```python
from build123d import *

# Parameters (mm, degrees)
F1_DEPTH = 63.5
F0_W     = 23.120732
F0_H     = 17.456719
F2_DEPTH = 25.4
F3_DEPTH = 7.9375
F5_R     = 6.35


with BuildPart() as f1:
    # F0 (on Front) → F1 (new body, symmetric)
    with BuildSketch(Plane.XZ):
        Polygon((23.818281, 9.525), (-41.275, 9.525), (-41.275, -9.525), (41.275, -9.525), (41.275, 9.525), align=None)
    extrude(amount=F1_DEPTH, both=True)

    # F0 (on Front) → F2 (join, symmetric)
    with BuildSketch(Plane.XZ):
        with Locations((71.885366, 61.128559)):
            Rectangle(F0_W, F0_H)
        with BuildLine():
            Line((23.818281, 36.5252), (23.818281, 9.525))
            Line((23.818281, 9.525), (41.275, 9.525))
            Line((41.275, 9.525), (41.275, 36.5252))
            ThreePointArc((41.275, 36.5252), (45.92468, 47.75052), (57.15, 52.4002))
            Line((57.15, 52.4002), (60.325, 52.4002))
            Line((60.325, 52.4002), (60.325, 69.856919))
            Line((60.325, 69.856919), (57.15, 69.856919))
            ThreePointArc((57.15, 69.856919), (33.580915, 60.094285), (23.818281, 36.5252))
        make_face()
    extrude(amount=F2_DEPTH, both=True)

    # F0 (on Front) → F3 (join, symmetric)
    with BuildSketch(Plane.XZ):
        with BuildLine():
            add(Edge.make_bspline(
                [(-41.275, 9.525), (-34.914378, 38.415078), (20.892713, 70.120394), (57.15, 69.856919)],
                knots=[0, 0, 0, 0, 115.44445, 115.44445, 115.44445, 115.44445], degree=3))
            Line((-41.275, 9.525), (23.818281, 9.525))
            Line((23.818281, 9.525), (23.818281, 36.5252))
            ThreePointArc((23.818281, 36.5252), (33.580915, 60.094285), (57.15, 69.856919))
        make_face()
    extrude(amount=F3_DEPTH, both=True)

    # F0 (on Front) → F4 (revolve)
    with BuildSketch(Plane.XZ):
        Polygon((83.445732, 76.2), (83.445732, 69.856919), (83.445732, 52.4002), (83.445732, 47.625), (111.125, 47.625), (111.125, 76.2), align=None)
    revolve(axis=Axis((83.445732, 0, 61.9125), (0, 0, 1)))

    # F5
    f5_edges = [f1.edges().sort_by_distance(p)[0] for p in [
        (-41.275, -63.5, 0),
        (41.275, -63.5, 0),
        (41.275, 63.5, 0),
        (-41.275, 63.5, 0),
    ]]
    fillet(f5_edges, radius=F5_R)


solid = f1.part
```
The model under review builds one solid part; all positions refer to its coordinate system, in mm. A direction names the side the tool comes from. Round coordinates to 2 decimals unless told otherwise and drop trailing zeros. Order: outer loops, then holes, each group sorted by start corner. A loop starts at its lowest first (then second) coordinate and runs counter-clockwise, first axis right, second up.
Item 1: Add section A-A, the plane y = -38. State the section outline as (x, z) points (3 decimals).
Working result:
outline: (-41.275, -9.525) - (41.275, -9.525) - (41.275, 9.525) - (-41.275, 9.525) - close
Item 2: Machinability: for faces 1 (the flat face through (64, -23, 52.4)), 2 (the flat face through (-2, -7.938, 33)), 3 (the flat face through (-2, 7.938, 33)), which of the approach directions +Z, -Z, +X, -X, +Y, -Y give a long, thin tool a straight path to every point of the face, cutting with its end or side? Answer none if there is none.
Working result:
face 1: -Z, -Y
face 2: +Z, -X, -Y
face 3: +Z, -X, +Y
Item 3: Add section B-B, the plane x = 89. State the section outline as (y, z) points (3 decimals).
Working result:
outline: (-27.116, 47.625) - (27.116, 47.625) - (27.116, 76.2) - (-27.116, 76.2) - close
Item 4: For pin 1 (5 mm diameter, centred on x = 64.5, y = 22.5, fed in from -Z) (3 decimals); pin 2 (1.6 mm diameter, centred on x = 58.5, y = 17, fed in from -Z); pin 3 (1 mm diameter, centred on x = 58.5, y = -15.5, fed in from +Z), all flat-tipped, find the tip position at first contact; note any pin that passes through.
Working result:
pin 1: stops at z = 47.625
pin 2: stops at z = 52.4
pin 3: stops at z = 69.86
Item 5: To check wall thickness, follow probe 1 along X at (y, z) = (8.5, -5) (3 decimals); probe 2 along Z at (x, y) = (-13.5, -30) (3 decimals); probe 3 along Y at (x, z) = (12, 39). State the ranges of each line that lie inside material, in increasing order.
Working result:
probe 1: x = -41.275 to 41.275
probe 2: z = -9.525 to 9.525
probe 3: y = -7.94 to 7.94
